Source: CAD feature listing. Evaluate the final solid. Frame: model axes, mm. Face numbers are marked on the shaded views. A direction names the side the tool comes from. Coordinates: 2 decimals unless noted, no trailing zeros. Order: outer loops, then holes, each group sorted by start corner. A loop starts at its lowest first (then second) coordinate and runs counter-clockwise, first axis right, second up.
Item 1: Ray query, line 1 (X direction, y = -0.5, z = -9); line 2 (Z direction, x = -17.5, y = 35.5); line 3 (Z direction, x = 73, y = -2). Return the intervals inside material, ascending.
Item 2: Contact query for flat-ended pins moving along their axis: P1, Ø6.5, axis at x = -41.49, z = 12.66, coming from the -Y side; P2, Ø5, axis at x = 57.74, z = -15.48, coming from the +Y side; P3, Ø1.3, axis at y = -24, z = 1, coming from the -X side; P4, Ø3, axis at x = 38.69, z = -26.48, coming from the +Y side. Output: stop coordinate, or through.
Item 3: Reachability of the marked faces 4 and 5 from +Z, -Z, +X, -X, +Y, -Y: full face, straight path, thin tool, end or side. Return the list, or none.
Item 4: Section B-B on x = 3.5. Return the cut outline in (y, z).
Item 5: Section A-A on y = 24. Return the cut outline in (x, z).
Item 6: Section D-D on z = -46.5. Return the cut outline in (x, y).
Item 7: Mould query, pull axis X, two halves, no side actions, for the marked faces 1, 2 and 3. Classes: released by +X, released by -X, zero draft, split by the parting line, or undercut.
Item 8: Section C-C on y = -39. State how many separate pieces and enclosed holes the cut face has, then the cut area to 3 significant figures.
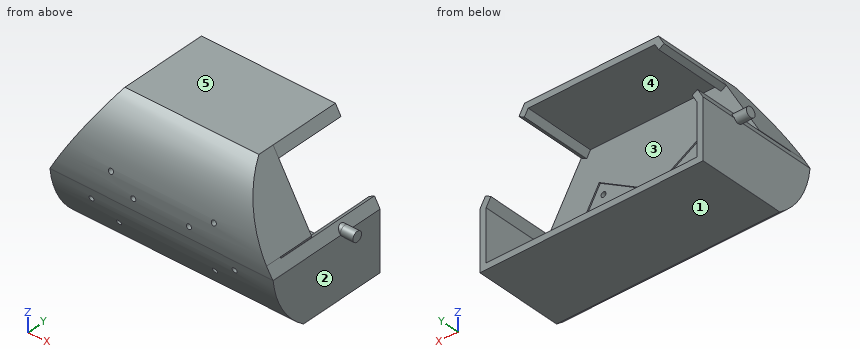
from build123d import *

# Parameters (mm, degrees)
BOSS_EXTRUDE1_DEPTH             = 50
BOSS_EXTRUDE1_DEPTH_BACK        = 50
CUT_EXTRUDE9_REACH              = 196.743
SHELL1_T                        = -5
SKETCH5_W                       = 54
SKETCH5_H                       = 87
CUT_EXTRUDE2_DEPTH              = 5
BOSS_EXTRUDE4_REACH             = 192.132
SKETCH6_R                       = 2
CUT_EXTRUDE4_DEPTH              = 121.370262108
SKETCH6_4_R                     = 2
CUT_EXTRUDE5_DEPTH              = 1
CUT_EXTRUDE10_REACH             = 122.37
SKETCH18_R                      = 4
BOSS_EXTRUDE5_DEPTH             = 10
BOSS_EXTRUDE5_DIRECTION_2_REACH = 196.743


with BuildPart() as part:
    # Sketch2 → Boss-Extrude1 (new, two sides: drawn at the far end of the back side and taken through both)
    with BuildSketch(Plane(origin=(0, 0, 0), x_dir=(1, 0, 0), z_dir=(0, 1, 0)).offset(-BOSS_EXTRUDE1_DEPTH_BACK)):
        Polygon((-90, 7.353829072), (-54, -55), (54, -55), (90, 7.353829072), (90, 55), (-90, 55), align=None)
    extrude(amount=BOSS_EXTRUDE1_DEPTH + BOSS_EXTRUDE1_DEPTH_BACK)

    # Sketch13 → Cut-Extrude9 (cut, up to next)
    with BuildSketch(Plane.ZY.offset(90), mode=Mode.PRIVATE) as cut_extrude9_sk1:
        with BuildLine():
            Line((-55, -21.268810449), (-55, -50))
            Line((-55, -50), (-7.353829072, -50))
            Line((-7.353829072, -50), (-7.353829072, -49.496068946))
            ThreePointArc((-7.353829072, -49.496068946), (-34.222719509, -40.523602958), (-55, -21.268810449))
        make_face()
    cut_extrude9_tool1 = extrude(cut_extrude9_sk1.sketch, amount=-CUT_EXTRUDE9_REACH, mode=Mode.PRIVATE) & part.part
    # Sketch13 → Cut-Extrude9 (cut, up to next)
    with BuildSketch(Plane.ZY.offset(90), mode=Mode.PRIVATE) as cut_extrude9_sk2:
        with BuildLine():
            Line((-7.353829072, -49.496068946), (-7.353829072, -50))
            Line((-7.353829072, -50), (55, -50))
            Line((55, -50), (55, -21.268810449))
            ThreePointArc((55, -21.268810449), (27.689960845, -43.924342078), (-7.353829072, -49.496068946))
        make_face()
    cut_extrude9_tool2 = extrude(cut_extrude9_sk2.sketch, amount=-CUT_EXTRUDE9_REACH, mode=Mode.PRIVATE) & part.part
    add(cut_extrude9_tool1.solids().sort_by_distance((-90, -41.817219, -41.87257))[0], mode=Mode.SUBTRACT)
    add(cut_extrude9_tool2.solids().sort_by_distance((-90, -41.875278, 41.569998))[0], mode=Mode.SUBTRACT)

    # Shell1
    shell1_openings = [part.faces().sort_by_distance(p)[0] for p in [
        (0, 50, -4.375017638),
    ]]
    offset(amount=SHELL1_T, openings=shell1_openings, kind=Kind.INTERSECTION)

    # Sketch5 → Cut-Extrude2 (cut)
    with BuildSketch(Plane(origin=(-64.315698604, 0, 37.132685902), x_dir=(0.500000000000001, 0, 0.8660254037844382), z_dir=(-0.866025403784438, 0, 0.5000000000000009))):
        with Locations((-15.368602792, 6.5)):
            Rectangle(SKETCH5_W, SKETCH5_H)
    cut_extrude2 = extrude(amount=-CUT_EXTRUDE2_DEPTH, mode=Mode.SUBTRACT)

    # Mirror1: Cut-Extrude2 across plane
    add(cut_extrude2.mirror(Plane(origin=(0, 0, 0), x_dir=(0, 0, 1), z_dir=(1, 0, 0))), mode=Mode.SUBTRACT)

    # Boss-Extrude4: up to this face of the body (flat: up to its plane)
    boss_extrude4_end = Plane(part.part.faces().sort_by_distance((85, 6.834453574, -28.402154485))[0])
    # Sketch16 → Boss-Extrude4 (add, up to the picked face)
    with BuildSketch(Plane(origin=(-85, 0, 0), x_dir=(0, 0, -1), z_dir=(1, 0, 0)), mode=Mode.PRIVATE) as boss_extrude4_sk1:
        with BuildLine():
            Line((-55, -8), (55, -8))
            Line((55, -8), (55, -21.268810449))
            ThreePointArc((55, -21.268810449), (0, -49.9), (-55, -21.268810449))
            Line((-55, -21.268810449), (-55, -8))
        make_face()
    boss_extrude4_tool1 = split(extrude(boss_extrude4_sk1.sketch, amount=BOSS_EXTRUDE4_REACH, mode=Mode.PRIVATE), bisect_by=boss_extrude4_end, keep=Keep.BOTH, mode=Mode.PRIVATE)
    add(boss_extrude4_tool1.solids().sort_by(Axis((-85, -25.669954, 0), (1, 0, 0)))[0])

    # Sketch6 → Cut-Extrude4 (cut, through all)
    with BuildSketch(Plane(origin=(0, -8, 0), x_dir=(1, 0, 0), z_dir=(0, 1, 0))):
        with Locations(Location((-57.742314098, 15.481878155, 0), (0, 0, 270))):
            Circle(SKETCH6_R)
        with Locations(Location((-38.689755215, 26.481878155, 0), (0, 0, 270))):
            Circle(SKETCH6_R)
        with Locations(Location((-41.492314098, -12.663947468, 0), (0, 0, 270))):
            Circle(SKETCH6_R)
        with Locations(Location((-22.439755215, -1.663947468, 0), (0, 0, 270))):
            Circle(SKETCH6_R)
        with Locations(Location((22.439755215, -1.663947468, 0), (0, 0, 56.302025246))):
            Circle(SKETCH6_R)
        with Locations(Location((41.492314098, -12.663947468, 0), (0, 0, 270))):
            Circle(SKETCH6_R)
        with Locations(Location((38.689755215, 26.481878155, 0), (0, 0, 270))):
            Circle(SKETCH6_R)
        with Locations(Location((57.742314098, 15.481878155, 0), (0, 0, 270))):
            Circle(SKETCH6_R)
    extrude(amount=-CUT_EXTRUDE4_DEPTH, mode=Mode.SUBTRACT)

    # Sketch6<4> → Cut-Extrude5 (cut)
    # profile 1 of 2: a face of its own
    with BuildSketch(Plane(origin=(0, -8, 0), x_dir=(1, 0, 0), z_dir=(0, 1, 0))):
        Polygon((36.127577388, 36.044055982), (67.304491924, 18.044055982), (44.054491924, -22.226125294), (12.877577388, -4.226125294), align=None)
        with Locations(Location((38.689755215, 26.481878155, 0), (0, 0, 270))):
            Circle(SKETCH6_4_R, mode=Mode.SUBTRACT)
        with Locations(Location((22.439755215, -1.663947468, 0), (0, 0, 270))):
            Circle(SKETCH6_4_R, mode=Mode.SUBTRACT)
        with Locations(Location((41.492314098, -12.663947468, 0), (0, 0, 270))):
            Circle(SKETCH6_4_R, mode=Mode.SUBTRACT)
        with Locations(Location((57.742314098, 15.481878155, 0), (0, 0, 270))):
            Circle(SKETCH6_4_R, mode=Mode.SUBTRACT)
    # profile 2 of 2: a face of its own
    with BuildSketch(Plane(origin=(0, -8, 0), x_dir=(1, 0, 0), z_dir=(0, 1, 0))):
        Polygon((-36.127577388, 36.044055982), (-12.877577388, -4.226125294), (-44.054491924, -22.226125294), (-67.304491924, 18.044055982), align=None)
    extrude(amount=-CUT_EXTRUDE5_DEPTH, mode=Mode.SUBTRACT)

    # Sketch17 → Cut-Extrude10 (cut, up to next)
    with BuildSketch(Plane(origin=(0, -8, 0), x_dir=(1, 0, 0), z_dir=(0, 1, 0)), mode=Mode.PRIVATE) as cut_extrude10_sk1:
        Polygon((-54, -55), (-85, -55), (-85, -1.306424965), align=None)
    cut_extrude10_tool1 = extrude(cut_extrude10_sk1.sketch, amount=-CUT_EXTRUDE10_REACH, mode=Mode.PRIVATE) & part.part
    # Sketch17 → Cut-Extrude10 (cut, up to next)
    with BuildSketch(Plane(origin=(0, -8, 0), x_dir=(1, 0, 0), z_dir=(0, 1, 0)), mode=Mode.PRIVATE) as cut_extrude10_sk2:
        Polygon((85, -55), (54, -55), (85, -1.306424965), align=None)
    cut_extrude10_tool2 = extrude(cut_extrude10_sk2.sketch, amount=-CUT_EXTRUDE10_REACH, mode=Mode.PRIVATE) & part.part
    add(cut_extrude10_tool1.solids().sort_by_distance((-74.666667, -8, 37.102142))[0], mode=Mode.SUBTRACT)
    add(cut_extrude10_tool2.solids().sort_by_distance((74.666667, -8, 37.102142))[0], mode=Mode.SUBTRACT)

    # Sketch18 → Boss-Extrude5 (add)
    with BuildSketch(Plane.ZY.offset(90)):
        with Locations((-5.755783353, 17.2426)):
            Circle(SKETCH18_R)
    boss_extrude5 = extrude(amount=BOSS_EXTRUDE5_DEPTH)

    # Sketch18 → Boss-Extrude5 direction 2 (add, up to next)
    with BuildSketch(Plane.ZY.offset(90), mode=Mode.PRIVATE) as boss_extrude5_direction_2_sk1:
        with Locations((-5.755783353, 17.2426)):
            Circle(SKETCH18_R)
    boss_extrude5_direction_2_tool1 = extrude(boss_extrude5_direction_2_sk1.sketch, amount=-BOSS_EXTRUDE5_DIRECTION_2_REACH, mode=Mode.PRIVATE) - part.part
    boss_extrude5_direction_2 = boss_extrude5_direction_2_tool1.solids().sort_by_distance((-90, 17.2426, -5.755783))[0]
    add(boss_extrude5_direction_2)

    # Mirror2: Boss-Extrude5, Boss-Extrude5 direction 2 across plane
    add(boss_extrude5.mirror(Plane(origin=(0, 0, 0), x_dir=(0, 0, 1), z_dir=(1, 0, 0))))
    add(boss_extrude5_direction_2.mirror(Plane(origin=(0, 0, 0), x_dir=(0, 0, 1), z_dir=(1, 0, 0))))


solid = part.part
Answer list:
1. line 1: x = -90 to -85, 85 to 90
1. line 2: z = -55 to -50, 50 to 55
1. line 3: z = -55 to -50
2. P1: stops at y = -49.24
2. P2: stops at y = -9
2. P3: stops at x = -85.55
2. P4: passes through
3. face 4: +Y
3. face 5: +Z, +X, -X, +Y, -Y
4. outline: (-21.27, -55) - (50, -55) - (50, -50) - (-8, -50) - (-8, 50) - (50, 50) - (50, 55) - (-21.27, 55) arc R67.14 ccw to start
5. outline: (-90, -55) - (90, -55) - (90, -7.35) - (85.5, 0.44) - (81.17, -2.06) - (85, -8.69) - (85, -50) - (-85, -50) - (-85, -8.69) - (-81.17, -2.06) - (-85.5, 0.44) - (-90, -7.35) - close; (-58.5, 47.21) - (-54.17, 44.71) - (-51.11, 50) - (51.11, 50) - (54.17, 44.71) - (58.5, 47.21) - (54, 55) - (-54, 55) - close
6. outline: (-90, -31.19) - (90, -31.19) - (90, 50) - (85, 50) - (85, -8) - (-85, -8) - (-85, 50) - (-90, 50) - close
7. face 1: zero draft
7. face 2: released by +X
7. face 3: undercut
8. separate pieces: 1
8. enclosed holes: 8
8. area: 12,000 mm2
